```python
from build123d import *

# Parameters (mm, degrees)
BOSS_EXTRUDE1_DEPTH = 70
FILLET1_R           = 10
SKETCH2_R           = 5
CUT_EXTRUDE1_DEPTH  = 10


with BuildPart() as part:
    # Sketch1 → Boss-Extrude1 (new body)
    with BuildSketch(Plane.XY):
        with BuildLine():
            Line((110.200913438, 15.404640081), (142.020718591, -16.415165072))
            ThreePointArc((142.020718591, -16.415165072), (143.720696939, -17.551054289), (145.725958124, -17.949925539))
            Line((145.725958124, -17.949925539), (171.583822501, -17.949925539))
            Line((171.583822501, -17.949925539), (171.583822501, -22.709925539))
            Line((171.583822501, -22.709925539), (145.725958124, -22.709925539))
            ThreePointArc((145.725958124, -22.709925539), (141.899123801, -21.948720864), (138.654890312, -19.780993351))
            Line((138.654890312, -19.780993351), (106.835085159, 12.038811802))
            ThreePointArc((106.835085159, 12.038811802), (103.590851671, 14.206539316), (99.764017347, 14.967743991))
            Line((99.764017347, 14.967743991), (12.581613091, 14.967743991))
            Line((12.581613091, 14.967743991), (-99.764017347, 14.967743991))
            ThreePointArc((-99.764017347, 14.967743991), (-103.590851671, 14.206539316), (-106.835085159, 12.038811802))
            Line((-106.835085159, 12.038811802), (-138.654890312, -19.780993351))
            ThreePointArc((-138.654890312, -19.780993351), (-141.899123801, -21.948720864), (-145.725958124, -22.709925539))
            Line((-145.725958124, -22.709925539), (-171.583822501, -22.709925539))
            Line((-171.583822501, -22.709925539), (-171.583822501, -17.949925539))
            Line((-171.583822501, -17.949925539), (-145.725958124, -17.949925539))
            ThreePointArc((-145.725958124, -17.949925539), (-143.720696939, -17.551054289), (-142.020718591, -16.415165072))
            Line((-142.020718591, -16.415165072), (-110.200913438, 15.404640081))
            ThreePointArc((-110.200913438, 15.404640081), (-105.412424809, 18.60420589), (-99.764017347, 19.727743991))
            Line((-99.764017347, 19.727743991), (12.581613091, 19.727743991))
            Line((12.581613091, 19.727743991), (99.764017347, 19.727743991))
            ThreePointArc((99.764017347, 19.727743991), (105.412424809, 18.60420589), (110.200913438, 15.404640081))
        make_face()
    extrude(amount=-BOSS_EXTRUDE1_DEPTH)

    # Fillet1
    fillet1_edges = [part.edges().sort_by_distance(p)[0] for p in [
        (171.583822501, -20.329925539, 0),
        (-171.583822501, -20.329925539, 0),
        (-171.583822501, -20.329925539, -70),
        (171.583822501, -20.329925539, -70),
    ]]
    fillet(fillet1_edges, radius=FILLET1_R)

    # Sketch2 → Cut-Extrude1 (cut)
    with BuildSketch(Plane(origin=(0, -17.949925539, 0), x_dir=(1, 0, 0), z_dir=(0, 1, 0))):
        with BuildLine():
            ThreePointArc((153.654890312, 53.854773815), (158.654890312, 48.854773815), (163.654890312, 53.854773815))
            Line((163.654890312, 53.854773815), (153.654890312, 53.854773815))
        make_face()
        with BuildLine():
            Line((153.654890312, 53.854773815), (163.654890312, 53.854773815))
            ThreePointArc((163.654890312, 53.854773815), (158.654890312, 58.854773815), (153.654890312, 53.854773815))
        make_face()
        with Locations(Location((158.654890312, 16.145226185, 0), (0, 0, 180))):
            Circle(SKETCH2_R)
    cut_extrude1 = extrude(amount=-CUT_EXTRUDE1_DEPTH, mode=Mode.SUBTRACT)

    # Mirror1: Cut-Extrude1 across plane
    add(cut_extrude1.mirror(Plane(origin=(0, 0, 0), x_dir=(0, 0, 1), z_dir=(1, 0, 0))), mode=Mode.SUBTRACT)


solid = part.part
```
For this review, take the finished solid that the model builds, in its own axes (mm). A direction names the side the tool comes from. Coordinates: 2 decimals unless noted, no trailing zeros. Loops run counter-clockwise (first coordinate to the right, second up) from the corner with the lowest first, then second, coordinate; pieces in that order, holes last.
1. Add section C-C, the plane x = 13. Give the boundary of the cut face in (y, z), then the cut area to 3 significant figures.
2. Mouldability with a two-part tool opening along X and no side actions: class faces 1 (the cylindrical face through (105.337, 18.635, -34.51)), 2 (the cylindrical face through (-160.96, -20.3, -49.42)), 3 (the cylindrical face through (-103.54, 14.227, -34.51)), 4 (the flat face through (1, 16, -70)) as +X half, -X half, draft (parallel to the pull), parting line (faces both ways), or undercut.
3. Add section A-A, the plane y = -1. Give the boundary of the cut face in (x, z), then the cut area to 3 significant figures.
4. Add section B-B, the plane z = -31. Give the boundary of the cut face in (x, y).
5. For faces 5 (the flat face through (159, -22.71, -35)), 6 (the cylindrical face through (-141.85, -21.93, -34.51)), list the 3-axis set-ups (+Z, -Z, +X, -X, +Y, -Y) from which the entire face can be reached by the end or side of a thin tool; tool diameter is ignored.
6. Add section D-D, the plane x = -132. Give the boundary of the cut face in (y, z).
7. For line 1 (Y direction, x = -74, z = -14.5); line 2 (X direction, y = 3, z = -44.5); line 3 (X direction, y = -13, z = -31), list the stretches that pass through material, from the lowest coordinate up.
8. Insertion check: P1, Ø6, axis at y = 11, z = -10, coming from the +X side; P2, Ø1.5, axis at x = 115.5, z = -23.5, coming from the +Y side; P3, Ø6, axis at x = 158.65, z = -16.15, coming from the -Y side; P4, Ø16, axis at x = -158.65, z = -53.85, coming from the +Y side. Each pin has a flat end and moves straight along its axis. Give the tip position at first contact, or say it passes through.
Result:
1. outline: (14.97, -70) - (19.73, -70) - (19.73, 0) - (14.97, 0) - close
1. area: 333 mm2
2. face 1: +X half
2. face 2: undercut
2. face 3: undercut
2. face 4: draft
3. outline: (-126.61, -70) - (-119.87, -70) - (-119.87, 0) - (-126.61, 0) - close; (119.87, -70) - (126.61, -70) - (126.61, 0) - (119.87, 0) - close
3. area: 942 mm2
4. outline: (-171.58, -22.71) - (-145.73, -22.71) arc R10 ccw to (-138.65, -19.78) - (-106.84, 12.04) arc R10 cw to (-99.76, 14.97) - (99.76, 14.97) arc R10 cw to (106.84, 12.04) - (138.65, -19.78) arc R10 ccw to (145.73, -22.71) - (171.58, -22.71) - (171.58, -17.95) - (145.73, -17.95) arc R5.24 cw to (142.02, -16.42) - (110.2, 15.4) arc R14.76 ccw to (99.76, 19.73) - (-99.76, 19.73) arc R14.76 ccw to (-110.2, 15.4) - (-142.02, -16.42) arc R5.24 cw to (-145.73, -17.95) - (-171.58, -17.95) - close
5. face 5: +Z, -Z, +X, -X, -Y
5. face 6: +Z, -Z, -Y
6. outline: (-13.13, -70) - (-6.39, -70) - (-6.39, 0) - (-13.13, 0) - close
7. line 1: y = 14.97 to 19.73
7. line 2: x = -122.61 to -115.87, 115.87 to 122.61
7. line 3: x = -138.61 to -131.87, 131.87 to 138.61
8. P1: stops at x = 117.61
8. P2: stops at y = 10.86
8. P3: passes through
8. P4: stops at y = -17.95
